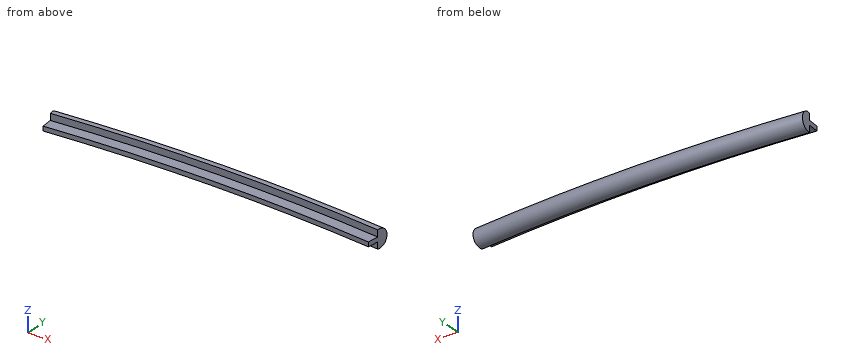
from build123d import *

# Parameters (mm, degrees)
REVOLVE1_ANGLE           = 5.229758018
REVOLVE1_OTHER_WAY_ANGLE = 5.229758018


with BuildPart() as part:
    # Sketch2 → Revolve1 (revolve)
    with BuildSketch(Plane(origin=(0, 0, 0), x_dir=(0, 0, -1), z_dir=(1, 0, 0))):
        with BuildLine():
            Line((0, 239.8), (0.3, 239.8))
            Line((0.3, 239.8), (0.3, 241.3))
            Line((0.3, 241.3), (1.18, 241.3))
            ThreePointArc((1.18, 241.3), (0, 242.800182019), (-1.18, 241.3))
            Line((-1.18, 241.3), (-0.3, 241.3))
            Line((-0.3, 241.3), (-0.3, 239.8))
            Line((-0.3, 239.8), (0, 239.8))
        make_face()
    revolve(axis=Axis((0, 0, 70.597641597), (0, 0, -1)), revolution_arc=REVOLVE1_ANGLE)

    # Sketch2 → Revolve1 other way (revolve)
    with BuildSketch(Plane(origin=(0, 0, 0), x_dir=(0, 0, -1), z_dir=(1, 0, 0))):
        with BuildLine():
            Line((0, 239.8), (0.3, 239.8))
            Line((0.3, 239.8), (0.3, 241.3))
            Line((0.3, 241.3), (1.18, 241.3))
            ThreePointArc((1.18, 241.3), (0, 242.800182019), (-1.18, 241.3))
            Line((-1.18, 241.3), (-0.3, 241.3))
            Line((-0.3, 241.3), (-0.3, 239.8))
            Line((-0.3, 239.8), (0, 239.8))
        make_face()
    revolve(axis=Axis((0, 0, 70.597641597), (0, 0, 1)), revolution_arc=REVOLVE1_OTHER_WAY_ANGLE)


solid = part.part
Here's how the part is built. I have some questions about the finished solid (model axes, mm). Coordinates: 2 decimals unless noted, no trailing zeros. Order: outer loops, then holes, each group sorted by start corner. A loop starts at its lowest first (then second) coordinate and runs counter-clockwise, first axis right, second up. Notation, with made-up numbers: M 51,58.5 L 67,58.5 A8 ccw 67,73.5 Z; hole C 32.25,11 d8. An arc over 180 degrees is marked long. Answer as CSV lines item,"result". Start each with the question number.
1. I need wall thicknesses on line 1 (Z direction, x = 17, y = 241.3); line 2 (Z direction, x = 13.5, y = 240); line 3 (Y direction, x = -19, z = -1). Which ranges of each line are inside material? Lowest first, please. Write a range as [from, to].
2. For pin 1 (1 mm diameter, centred on y = 241, z = 0.5, fed in from -X); pin 2 (2 mm diameter, centred on x = 5, y = 240, fed in from -Z); pin 3 (1.2 mm diameter, centred on x = -8, y = 239.5, fed in from +Z), each with a flat end and sliding along its axis, tell me the tip position at first contact or that it passes through.
3. I want a section at B-B, the plane z = -0.7. Write out the boundary of the cut face in (x, y), and give its area (3 significant figures).
4. I want a section at A-A, the plane y = 239.2. Write out the boundary of the cut face in (x, z), and give its area (3 significant figures).
Recorded:
1,line 1,"z = [-1.17, 1.17]"
1,line 2,"z = [-0.3, 0.3]"
1,line 3,"y = [240.55, 241.53]"
2,pin 1,"stops at x = -22.1"
2,pin 2,"stops at z = -0.3"
2,pin 3,"stops at z = 0.3"
3,outline,"M -22.11,241.57 L -21.99,240.3 A241.3 cw 21.99,240.3 L 22.11,241.57 A242.58 ccw Z"
3,area,"56.4 mm2"
4,outline,"M -21.89,-0.3 L -16.95,-0.3 L -16.95,0.3 L -21.89,0.3 Z; M 16.95,-0.3 L 21.89,-0.3 L 21.89,0.3 L 16.95,0.3 Z"
4,area,"5.93 mm2"
